```python
from build123d import *

# Parameters (mm, degrees)
AUFSATZ_LINEAR_START            = 170
AUFSATZ_LINEAR_AUSTRAGEN1_DEPTH = 35
SKIZZE6_R                       = 4
SCHNITT_LINEAR_AUSTRAGEN1_DEPTH = 21


with BuildPart() as part:
    # Skizze4 → Aufsatz-Linear austragen1 (new body)
    with BuildSketch(Plane(origin=(0, 0, 0), x_dir=(1, 0, 0), z_dir=(0, 1, 0)).offset(AUFSATZ_LINEAR_START)):
        Polygon((25.15, -12.65), (33.5, -12.65), (33.5, 21), (-25.25, 21), (-25.25, 12.65), (25.15, 12.65), align=None)
    extrude(amount=AUFSATZ_LINEAR_AUSTRAGEN1_DEPTH)

    # Skizze6 → Schnitt-Linear austragen1 (cut)
    with BuildSketch(Plane.XY):
        with Locations((-13.5, 190)):
            Circle(SKIZZE6_R)
        with Locations((13.5, 190)):
            Circle(SKIZZE6_R)
    extrude(amount=-SCHNITT_LINEAR_AUSTRAGEN1_DEPTH, mode=Mode.SUBTRACT)


solid = part.part
```
Work out the finished part from the listing and answer in its coordinate system (mm). A direction names the side the tool comes from. Give positions to 0.01 mm unless a question says otherwise; leave off trailing zeros. Loops run counter-clockwise (first coordinate to the right, second up) from the corner with the lowest first, then second, coordinate; pieces in that order, holes last. Notation, with made-up numbers: (20, -27) -> (72, -27) arc R7 cw to (72, -20) -> close; hole circle Ø3 at (21.25, 68.25). An arc over 180 degrees is marked (long way). Put each result on its own line as item: value. Start each with the question number.
Item 1: The part is cut by section B-B (x = -15). Give the vertices of the cut face in (y, z), then the cut area to 3 significant figures.
Item 2: The part is cut by section C-C (z = -18). Give the vertices of the cut face in (x, y), then the cut area to 3 significant figures.
Item 3: Which of the six approach directions +Z, -Z, +X, -X, +Y, -Y give full straight-line access (tool end or side, diameter ignored) to faces 4 (the face through (12.979, 193.966, -16.767)), 5 (the face through (25.15, 187, 0))?
Item 4: The part is cut by section D-D (y = 178). Give the vertices of the cut face in (x, z), then the cut area to 3 significant figures.
Item 5: The part is cut by section A-A (y = 190). Give the vertices of the cut face in (x, z).
Item 6: Each of these flat-tipped pins is pushed along its axis until it touches: P1, Ø1, axis at y = 175.5, z = -7, coming from the -X side; P2, Ø3, axis at x = -17.5, z = -11, coming from the +Y side; P3, Ø4, axis at x = -11.5, y = 186.5, coming from the +Z side. Where does it stop, or does it pass through?
Item 7: The mould has two halves that part along X. Classify faces 1 (the face through (33.5, 187, -4)), 2 (the face through (0, 187, -12.65)), 3 (the face through (-14.021, 193.966, -16.767)): released by +X, released by -X, zero draft, split by the parting line, or undercut.
Item 8: Find the intervals of material crossed by L1, parallel to Y at x = 13.5, z = -15; L2, parallel to Z at x = 8, y = 185; L3, parallel to X at y = 187.5, z = -16.5, in increasing order. Write a range as [from, to].
Answers below:
1. outline: (170, -21) -> (186.29, -21) -> (186.29, -12.65) -> (170, -12.65) -> close; (193.71, -21) -> (205, -21) -> (205, -12.65) -> (193.71, -12.65) -> close
1. area: 230 mm2
2. outline: (-25.25, 170) -> (33.5, 170) -> (33.5, 205) -> (-25.25, 205) -> close; hole circle Ø8 at (-13.5, 190); hole circle Ø8 at (13.5, 190)
2. area: 1,960 mm2
3. face 4: +Z, -Z
3. face 5: +Z, -X, +Y, -Y
4. outline: (-25.25, -21) -> (33.5, -21) -> (33.5, 12.65) -> (25.15, 12.65) -> (25.15, -12.65) -> (-25.25, -12.65) -> close
4. area: 702 mm2
5. outline: (-25.25, -21) -> (-17.5, -21) -> (-17.5, -12.65) -> (-25.25, -12.65) -> close; (-9.5, -21) -> (9.5, -21) -> (9.5, -12.65) -> (-9.5, -12.65) -> close; (17.5, -21) -> (33.5, -21) -> (33.5, 12.65) -> (25.15, 12.65) -> (25.15, -12.65) -> (17.5, -12.65) -> close
6. P1: x = 25.15
6. P2: through
6. P3: z = -12.65
7. face 1: released by +X
7. face 2: zero draft
7. face 3: undercut
8. L1: [170, 186], [194, 205]
8. L2: [-21, -12.65]
8. L3: [-25.25, -16.62], [-10.38, 10.38], [16.62, 33.5]
